Part model, mm, in its own coordinate system. A direction names the side the tool comes from. Give positions to 0.01 mm unless a question says otherwise; leave off trailing zeros. Write each loop counter-clockwise with the first axis right and the second up, starting at its lowest first coordinate (ties: lowest second). Pieces come first, ordered by that corner, then holes. Notation, with made-up numbers: M -28.75,56 L 26.25,56 A15 ccw 26.25,79 Z; hole C 29,-36 d1. An arc over 180 degrees is marked long. Answer as CSV lines item,"result". Start each with the question number.
Item 1: Wall check: L1, parallel to X at y = 9.7, z = 0.3; L2, parallel to Y at x = 5.75, z = -0.25; L3, parallel to Z at x = -6, y = 3. Give the ranges that are in metal, low to high. Write a range as from..to.
Item 2: Band-saw the part on A-A, the plane z = 0.3. List the corners of the cut face in (x, y), then the cut area to 3 significant figures.
Item 3: Band-saw the part on D-D, the plane x = -6. List the corners of the cut face in (y, z).
Item 4: Band-saw the part on C-C, the plane y = 7. List the corners of the cut face in (x, z).
Item 5: Band-saw the part on B-B, the plane x = 0. List the corners of the cut face in (y, z).
Item 6: 3-axis set-ups, long thin cutter, end or side, ignore diameter. For faces 1 (the flat face through (5, 2, -3.7)), 2 (the cylindrical face through (-6.75, 9.75, 0.22)), 3 (the flat face through (0, 5.8, -4)): which of +Z, -Z, +X, -X, +Y, -Y reach the whole face in a straight line?
Item 7: Pin check, flat tips, straight feed: pin 1 (1.6 mm diameter, centred on x = 4.5, y = 2.5, fed in from -Z); pin 2 (0.6 mm diameter, centred on x = -5, z = -4, fed in from +Y); pin 3 (5 mm diameter, centred on x = 4, y = 8.5, fed in from +Z). Stop position of each tip, or through.
Item 8: Two-plate mould, pull along X, no slides. Class faces 4 (the flat face through (7.5, 5, 0)), 5 (the cylindrical face through (-1.75, 9.75, 0.22)), 6 (the flat face through (-0.1, 7.9, -2.7)): +X half, -X half, draft (parallel to the pull), parting line (faces both ways), or undercut.
from build123d import *

# Parameters (mm, degrees)
SKETCH3_W           = 15
SKETCH3_H           = 8.4
BOSS_EXTRUDE3_DEPTH = 10
CUT_EXTRUDE1_DEPTH  = 16
SKETCH5_R           = 1.75
CUT_EXTRUDE2_DEPTH  = 0.5
SKETCH6_W           = 3
SKETCH6_H           = 2
CUT_EXTRUDE4_DEPTH  = 0.5
LPATTERN2_COUNT     = 3
LPATTERN2_PITCH     = 5


with BuildPart() as part:
    # Sketch3 → Boss-Extrude3 (new body)
    with BuildSketch(Plane(origin=(0, 0, 0), x_dir=(1, 0, 0), z_dir=(0, 1, 0))):
        Rectangle(SKETCH3_W, SKETCH3_H)
    extrude(amount=BOSS_EXTRUDE3_DEPTH)

    # Sketch4 → Cut-Extrude1 (cut, through all)
    with BuildSketch(Plane.ZY.offset(7.5)):
        Polygon((-3.4, 5.8), (-2, 10), (-3.4, 10), (-4.2, 10), (-4.2, 5.8), align=None)
        Polygon((4.2, 10), (2.6, 10), (4.2, 4), align=None)
    extrude(amount=-CUT_EXTRUDE1_DEPTH, mode=Mode.SUBTRACT)

    # Sketch5 → Cut-Extrude2 (cut)
    with BuildSketch(Plane(origin=(0, 10, 0), x_dir=(1, 0, 0), z_dir=(0, 1, 0))):
        with Locations((-5, -0.3)):
            Circle(SKETCH5_R)
    cut_extrude2 = extrude(amount=-CUT_EXTRUDE2_DEPTH, mode=Mode.SUBTRACT)

    # Sketch6 → Cut-Extrude4 (cut)
    with BuildSketch(Plane(origin=(0, 0, -4.2), x_dir=(-1, 0, 0), z_dir=(0, 0, -1))):
        with Locations((5, 2.4)):
            Rectangle(SKETCH6_W, SKETCH6_H)
    cut_extrude4 = extrude(amount=-CUT_EXTRUDE4_DEPTH, mode=Mode.SUBTRACT)

    # LPattern2: Cut-Extrude2, Cut-Extrude4 ×3
    with Locations(*[(i * LPATTERN2_PITCH, 0, 0) for i in range(1, LPATTERN2_COUNT)]):
        add(cut_extrude2, mode=Mode.SUBTRACT)
        add(cut_extrude4, mode=Mode.SUBTRACT)


solid = part.part
Output:
1,L1,"-7.5..-6.75, -3.25..-1.75, 1.75..3.25, 6.75..7.5"
1,L2,"0..9.5"
1,L3,"-3.7..4.2"
2,outline,"M -7.5,0 L 7.5,0 L 7.5,10 L 6.75,10 L 6.75,9.5 L 3.25,9.5 L 3.25,10 L 1.75,10 L 1.75,9.5 L -1.75,9.5 L -1.75,10 L -3.25,10 L -3.25,9.5 L -6.75,9.5 L -6.75,10 L -7.5,10 Z"
2,area,"145 mm²"
3,outline,"M 0,-4.2 L 1.4,-4.2 L 1.4,-3.7 L 3.4,-3.7 L 3.4,-4.2 L 5.8,-4.2 L 5.8,-3.4 L 10,-2 L 10,-1.14 L 9.5,-1.14 L 9.5,1.74 L 10,1.74 L 10,2.6 L 4,4.2 L 0,4.2 Z"
4,outline,"M -7.5,-3 L 7.5,-3 L 7.5,3.4 L -7.5,3.4 Z"
5,outline,"M 0,-4.2 L 1.4,-4.2 L 1.4,-3.7 L 3.4,-3.7 L 3.4,-4.2 L 5.8,-4.2 L 5.8,-3.4 L 10,-2 L 10,-1.45 L 9.5,-1.45 L 9.5,2.05 L 10,2.05 L 10,2.6 L 4,4.2 L 0,4.2 Z"
6,face 1,"-Z"
6,face 2,"+Y"
6,face 3,"-Z, +X, -X, +Y"
7,pin 1,"z = -3.7"
7,pin 2,"y = 5.8"
7,pin 3,"z = 3.67"
8,face 4,"+X half"
8,face 5,"undercut"
8,face 6,"draft"
